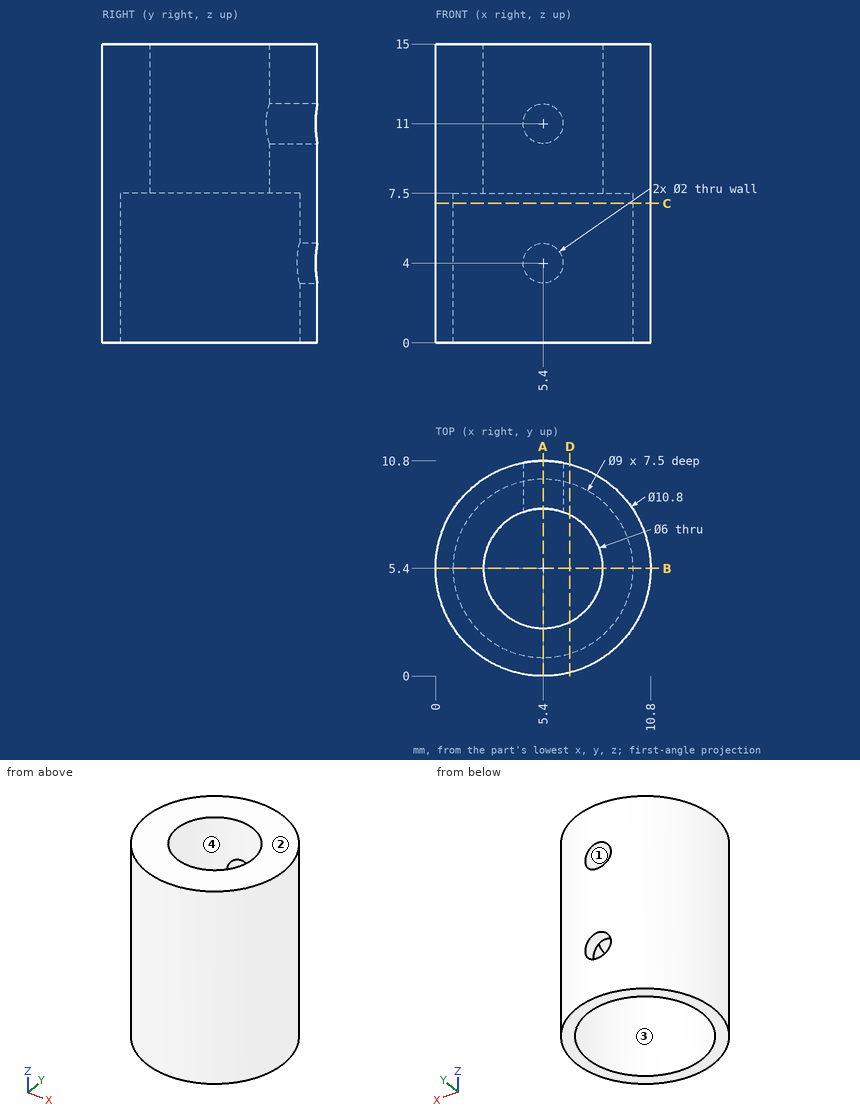
Can you work these out from the drawing? Everything is in mm from the part's minimum corner. A direction names the side the tool comes from. Round coordinates to 2 decimals unless told otherwise and drop trailing zeros. Loops run counter-clockwise (first coordinate to the right, second up) from the corner with the lowest first, then second, coordinate; pieces in that order, holes last. Notation, with made-up numbers: (46, 45) - (84, 45) arc R17 cw to (84, 76) - close; hole circle Ø3 at (-13, -23). An arc over 180 degrees is marked (long way). Answer in a Markdown table with one row per item. Add a question column.
(1) If we section it at A-A (x = 5.4): Please give me the cut outline in (y, z), plus the area to 3 significant figures.
(2) If we section it at C-C (z = 7): Please give me the cut outline in (x, y), plus the area to 3 significant figures.
(3) For the marked faces 3 and 4, which set-ups out of +Z, -Z, +X, -X, +Y, -Y let a thin tool reach every point of the face, with its end or its side?
(4) If we section it at D-D (x = 6.75): Please give me the cut outline in (y, z), plus the area to 3 significant figures.
(5) If we section it at B-B (y = 5.4): Please give me the cut outline in (x, z), plus the area to 3 significant figures.
(6) I'm going to push flat-ended pins straight in: pin 1 (6 mm diameter, centred on y = 9.5, z = 10.5, fed in from -X); pin 2 (2.5 mm diameter, centred on x = 5.4, z = 4, fed in from +Y); pin 3 (5 mm diameter, centred on x = 2, z = 2, fed in from +Y); pin 4 (5 mm diameter, centred on x = 8.5, z = 2.5, fed in from -Y). Where does each tip first touch, or does it pass through?
(7) I need wall thicknesses on line 1 along X through (y, z) = (5.5, 11.5); line 2 along Y through (x, z) = (5.4, 2.75); line 3 along Y through (x, z) = (3.5, 14.5). Which ranges of each line are inside material? Lowest first, please.
(8) If we mould it in two halves opening along Z, with no side actions, what happens to the marked faces 1 and 2? For each: pulls with the +Z half, pulls with the -Z half, needs draft (parallel to the pull), parting line crosses it, or undercut.
Model answer:
| question | item | result |
|---|---|---|
| 1 | outline | (0, 0) - (0.9, 0) - (0.9, 7.5) - (2.4, 7.5) - (2.4, 15) - (0, 15) - close; (8.4, 7.5) - (9.9, 7.5) - (9.9, 5) - (10.8, 5) - (10.8, 10) - (8.4, 10) - close; (8.4, 12) - (10.8, 12) - (10.8, 15) - (8.4, 15) - close; (9.9, 0) - (10.8, 0) - (10.8, 3) - (9.9, 3) - close |
| 1 | area | 42.9 mm² |
| 2 | outline | circle Ø10.8 at (5.4, 5.4); hole circle Ø9 at (5.4, 5.4) |
| 2 | area | 28.0 mm² |
| 3 | face 3 | -Z |
| 3 | face 4 | +Z, -Z |
| 4 | outline | (0.17, 0) - (1.11, 0) - (1.11, 7.5) - (2.72, 7.5) - (2.72, 15) - (0.17, 15) - close; (8.08, 7.5) - (9.69, 7.5) - (9.69, 0) - (10.63, 0) - (10.63, 15) - (8.08, 15) - close |
| 4 | area | 52.3 mm² |
| 5 | outline | (0, 0) - (0.9, 0) - (0.9, 7.5) - (2.4, 7.5) - (2.4, 15) - (0, 15) - close; (8.4, 7.5) - (9.9, 7.5) - (9.9, 0) - (10.8, 0) - (10.8, 15) - (8.4, 15) - close |
| 5 | area | 49.5 mm² |
| 6 | pin 1 | stops at x = 0.11 |
| 6 | pin 2 | stops at y = 10.8 |
| 6 | pin 3 | stops at y = 10.72 |
| 6 | pin 4 | stops at y = 0.03 |
| 7 | line 1 | x = 0 to 2.4, 8.4 to 10.8 |
| 7 | line 2 | y = 0 to 0.9, 9.9 to 10.8 |
| 7 | line 3 | y = 0.35 to 3.08, 7.72 to 10.45 |
| 8 | face 1 | undercut |
| 8 | face 2 | pulls with the +Z half |
